For this review, use the dimensioned drawing (mm, ordinates from the lowest corner) and the shaded views. A direction names the side the tool comes from. Coordinates: 2 decimals unless noted, no trailing zeros. Loops run counter-clockwise (first coordinate to the right, second up) from the corner with the lowest first, then second, coordinate; pieces in that order, holes last. Notation, with made-up numbers: (-10.5, 24) - (14.5, 24) arc R19 ccw to (14.5, 47) - close; hole circle Ø7 at (6.25, 44.25). An arc over 180 degrees is marked (long way). Use one line per item in the form item = value. Start each with the question number.
(1) Tool access review of the marked faces 4, 5, 6 and 7: name each direction out of +Z, -Z, +X, -X, +Y, -Y from which nothing blocks a thin tool from reaching the whole face with its end or side.
(2) Add section A-A (x = 15.75). State the section outline as (y, z) points.
(3) For L1, parallel to X at y = 8.5, z = 1.25; L2, parallel to X at y = 13.75, z = 6.25; L3, parallel to Y at x = 11.25, z = 6, list the stretches that pass through material, from the lowest coordinate up.
(4) Add section D-D (x = 1.5). State the section outline as (y, z) points (3 decimals), plus the area to 3 significant figures.
(5) Add section C-C (y = 10.75). State the section outline as (x, z) points.
(6) The part is to be moulded in two halves that separate along Y. For the marked faces 1, 2 and 3, say which applies: pulls with the +Y half, pulls with the -Y half, needs draft (parallel to the pull), parting line crosses it, or undercut.
(7) Add section B-B (z = 6.75). State the section outline as (x, y) points.
(8) Clearance check with flat-ended pins moving along their axes: pin 1 Ø5 at (x, y) = (9.5, 4) entering from -Z; pin 2 Ø0.6 at (x, y) = (4.5, 1.5) entering from -Z; pin 3 Ø1 at (x, z) = (14.5, 5.5) entering from +Y. State where each tip first meets the part, or that it passes through.
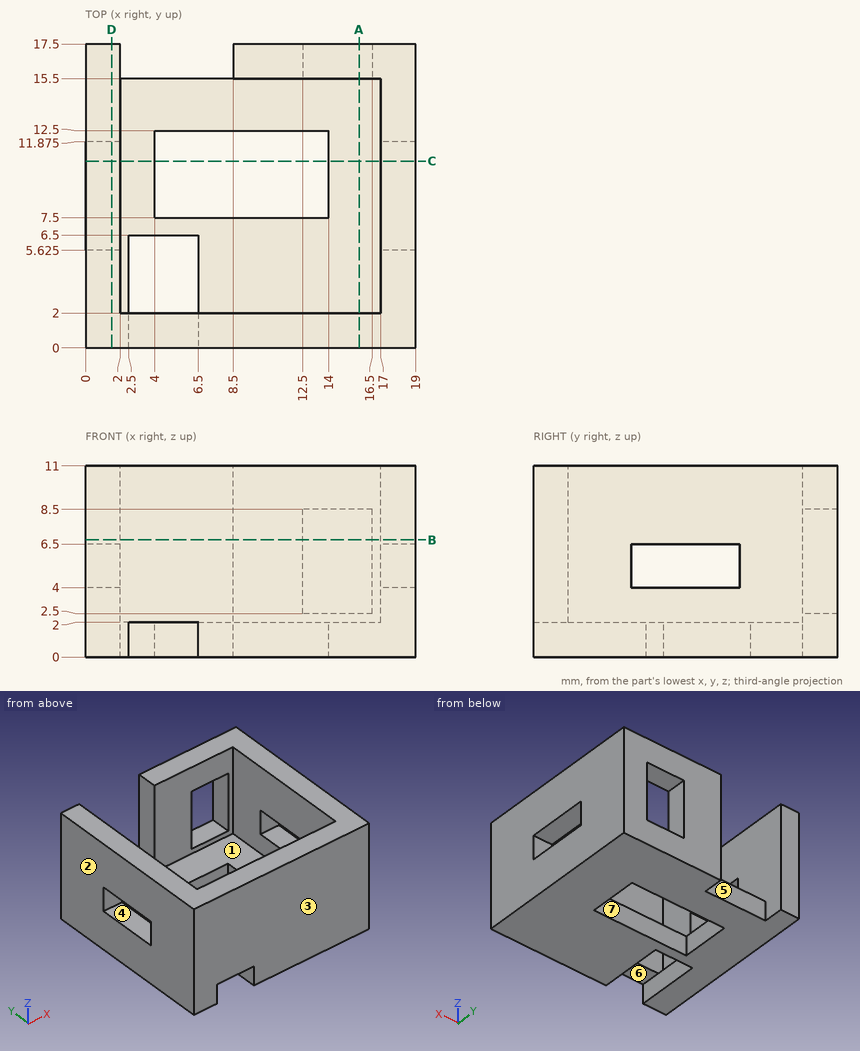
Computed values:
q1.face_4 = +X, -X
q1.face_5 = +Z, -Z, +Y
q1.face_6 = -Z, -Y
q1.face_7 = +Z, -Z
q2.outline = (0, 0) - (17.5, 0) - (17.5, 2.5) - (15.5, 2.5) - (15.5, 2) - (2, 2) - (2, 11) - (0, 11) - close; (15.5, 8.5) - (17.5, 8.5) - (17.5, 11) - (15.5, 11) - close
q3.L1 = 0 to 4, 14 to 19
q3.L2 = 0 to 2, 17 to 19
q3.L3 = 0 to 2, 15.5 to 17.5
q4.outline = (0, 0) - (17.5, 0) - (17.5, 11) - (0, 11) - close; hole (5.625, 4) - (11.875, 4) - (11.875, 6.5) - (5.625, 6.5) - close
q4.area = 177 mm^2
q5.outline = (0, 0) - (4, 0) - (4, 2) - (2, 2) - (2, 4) - (0, 4) - close; (0, 6.5) - (2, 6.5) - (2, 11) - (0, 11) - close; (14, 0) - (19, 0) - (19, 4) - (17, 4) - (17, 2) - (14, 2) - close; (17, 6.5) - (19, 6.5) - (19, 11) - (17, 11) - close
q6.face_1 = undercut
q6.face_2 = needs draft
q6.face_3 = pulls with the -Y half
q7.outline = (0, 0) - (19, 0) - (19, 17.5) - (16.5, 17.5) - (16.5, 15.5) - (17, 15.5) - (17, 2) - (2, 2) - (2, 17.5) - (0, 17.5) - close; (8.5, 15.5) - (12.5, 15.5) - (12.5, 17.5) - (8.5, 17.5) - close
q8.pin_1 = 0
q8.pin_2 = 2
q8.pin_3 = 2
